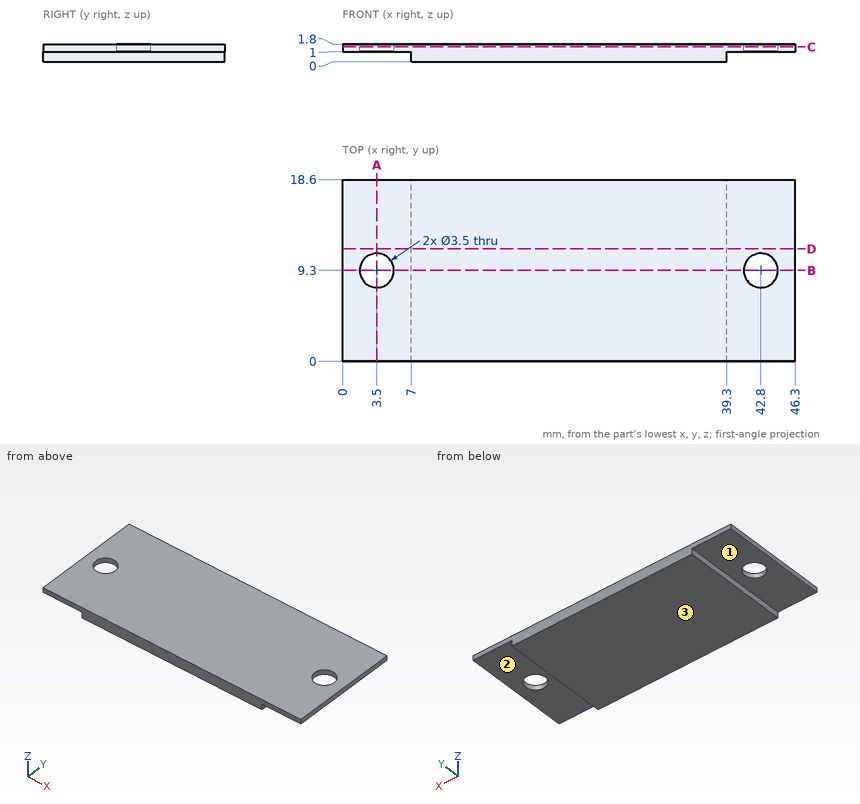
Input: dimensioned drawing with shaded views. Units: mm. Origin: part minimum x, y, z. A direction names the side the tool comes from. Coordinates: 2 decimals unless noted, no trailing zeros. Loops run counter-clockwise (first coordinate to the right, second up) from the corner with the lowest first, then second, coordinate; pieces in that order, holes last. Notation, with made-up numbers: (49.5, 62) -> (107.5, 62) arc R12 cw to (107.5, 73) -> close; hole circle Ø6 at (-37.75, -1.5). An arc over 180 degrees is marked (long way). One line per item, written item: value. Start each with the question number.
Q1. Line query: line 1 along Y through (x, z) = (42.8, 1.5); line 2 along X through (y, z) = (7.75, 1.35); line 3 along X through (y, z) = (8.75, 0.9). Output: solid intervals per line, ascending.
Q2. Section query C-C, the plane z = 1.5. Return the cut outline in (x, y).
Q3. Contact query for flat-ended pins moving along their axis: P1, Ø2, axis at x = 3.5, y = 9.3, coming from the +Z side (3 decimals); P2, Ø4.5, axis at x = 42.8, y = 9.3, coming from the -Z side. Output: stop coordinate, or through.
Q4. Section query B-B, the plane y = 9.3. Return the cut outline in (x, z).
Q5. Section query A-A, the plane x = 3.5. Return the cut outline in (y, z).
Q6. Set-up query: the marked faces 1, 2 and 3. Return all of +Z, -Z, +X, -X, +Y, -Y with unobstructed straight access to the full face (end or side cutting, diameter ignored); none if empty.
Q7. Section query D-D, the plane y = 11.5. Return the cut outline in (x, z).
Results:
1. line 1: 0 to 7.55, 11.05 to 18.6
1. line 2: 0 to 2.69, 4.31 to 41.99, 43.61 to 46.3
1. line 3: 7 to 39.3
2. outline: (0, 0) -> (46.3, 0) -> (46.3, 18.6) -> (0, 18.6) -> close; hole circle Ø3.5 at (3.5, 9.3); hole circle Ø3.5 at (42.8, 9.3)
3. P1: through
3. P2: z = 1
4. outline: (0, 1) -> (1.75, 1) -> (1.75, 1.8) -> (0, 1.8) -> close; (5.25, 1) -> (7, 1) -> (7, 0) -> (39.3, 0) -> (39.3, 1) -> (41.05, 1) -> (41.05, 1.8) -> (5.25, 1.8) -> close; (44.55, 1) -> (46.3, 1) -> (46.3, 1.8) -> (44.55, 1.8) -> close
5. outline: (0, 1) -> (7.55, 1) -> (7.55, 1.8) -> (0, 1.8) -> close; (11.05, 1) -> (18.6, 1) -> (18.6, 1.8) -> (11.05, 1.8) -> close
6. face 1: -Z, -X, +Y, -Y
6. face 2: -Z, +X, +Y, -Y
6. face 3: -Z, +X, -X, +Y, -Y
7. outline: (0, 1) -> (7, 1) -> (7, 0) -> (39.3, 0) -> (39.3, 1) -> (46.3, 1) -> (46.3, 1.8) -> (0, 1.8) -> close
